Check sheet for the modelled part. Datum: model origin and axes. Units: mm. Face numbers are marked on the shaded views. A direction names the side the tool comes from. Coordinates: 2 decimals unless noted, no trailing zeros. Order: outer loops, then holes, each group sorted by start corner. A loop starts at its lowest first (then second) coordinate and runs counter-clockwise, first axis right, second up.
from build123d import *

# Parameters (mm, degrees)
BOSS_EXTRUDE1_DEPTH  = 26.75
BOSS_EXTRUDE2_DEPTH  = 1.25
FILLET1_R            = 1.25
FILLET1_OF_MIRROR1_R = 1.25
SKETCH5_R            = 3
CUT_EXTRUDE1_DEPTH   = 1.25
SKETCH6_R            = 3
CUT_EXTRUDE2_DEPTH   = 1.25
CUT_EXTRUDE3_DEPTH   = 1.25
CUT_EXTRUDE4_DEPTH   = 1.25


with BuildPart() as part:
    # Sketch1 → Boss-Extrude1 (new body)
    with BuildSketch(Plane(origin=(0, 0, 0), x_dir=(0, 0, -1), z_dir=(1, 0, 0))):
        Polygon((45.443853174, 24.716321972), (-44.407308019, 15.814225038), (-85.72558755, -16.072016683), (-86.489274142, -15.082429501), (-44.887235053, 17.022795826), (45.320611525, 25.960231734), align=None)
    extrude(amount=BOSS_EXTRUDE1_DEPTH)

    # Sketch2 → Boss-Extrude2 (add)
    with BuildSketch(Plane(origin=(26.75, 0, 0), x_dir=(0, 0, -1), z_dir=(1, 0, 0))):
        Polygon((46.306544717, 16.008953638), (-41.047818784, 7.354229524), (-80.379781408, -22.999126953), (-86.489274142, -15.082429501), (-44.887235053, 17.022795826), (45.320611525, 25.960231734), align=None)
    boss_extrude2 = extrude(amount=BOSS_EXTRUDE2_DEPTH)

    # Fillet1
    fillet1_edges = [part.edges().sort_by_distance(p)[0] for p in [
        (28, 21.49151378, -0.216688236),
        (28, 0.970183162, 65.688254597),
    ]]
    fillet(fillet1_edges, radius=FILLET1_R)

    # Mirror1: Boss-Extrude2 across plane
    add(boss_extrude2.mirror(Plane(origin=(13.375, 0, 0), x_dir=(0, 0, 1), z_dir=(1, 0, 0))))

    # Fillet1 of Mirror1
    fillet1_of_mirror1_edges = [part.edges().sort_by_distance(p)[0] for p in [
        (-1.25, 21.49151378, -0.216688236),
        (-1.25, 0.970183162, 65.688254597),
    ]]
    fillet(fillet1_of_mirror1_edges, radius=FILLET1_OF_MIRROR1_R)

    # Sketch5 → Cut-Extrude1 (cut)
    with BuildSketch(Plane(origin=(0, 21.261342533, 2.106489551), x_dir=(1, 0, 0), z_dir=(0, 0.9951278095775022, 0.09859331927408967))):
        with Locations(Location((5.55625, 41.309306291, 0), (0, 0, 270))):
            Circle(SKETCH5_R)
        with Locations(Location((21.19375, 41.309306291, 0), (0, 0, 270))):
            Circle(SKETCH5_R)
    extrude(amount=-CUT_EXTRUDE1_DEPTH, mode=Mode.SUBTRACT)

    # Sketch6 → Cut-Extrude2 (cut)
    with BuildSketch(Plane(origin=(0, 32.379495301, 24.987981728), x_dir=(1, 0, 0), z_dir=(0, 0.7916697451364806, 0.6109492733734446))):
        with Locations(Location((21.19375, -71.335540962, 0), (0, 0, 270))):
            Circle(SKETCH6_R)
        with Locations(Location((5.55625, -71.335540962, 0), (0, 0, 270))):
            Circle(SKETCH6_R)
        with Locations(Location((5.55625, -46.335540962, 0), (0, 0, 270))):
            Circle(SKETCH6_R)
        with Locations(Location((21.19375, -46.335540962, 0), (0, 0, 270))):
            Circle(SKETCH6_R)
    extrude(amount=-CUT_EXTRUDE2_DEPTH, mode=Mode.SUBTRACT)

    # Sketch7 → Cut-Extrude3 (cut)
    with BuildSketch(Plane(origin=(0, 21.261342533, 2.106489551), x_dir=(1, 0, 0), z_dir=(0, 0.9951278095775022, 0.09859331927408967))):
        with BuildLine():
            Line((8.875, -42.943848047), (17.875, -42.943848047))
            Line((17.875, -42.943848047), (17.875, -38.104983203))
            ThreePointArc((17.875, -38.104983203), (17.435660172, -37.044323031), (16.375, -36.604983203))
            Line((16.375, -36.604983203), (10.375, -36.604983203))
            ThreePointArc((10.375, -36.604983203), (9.314339828, -37.044323031), (8.875, -38.104983203))
            Line((8.875, -38.104983203), (8.875, -42.943848047))
        make_face()
        with BuildLine():
            Line((17.875, -23.604983203), (17.875, -15.104983203))
            Line((17.875, -15.104983203), (17.875, -13.604983203))
            ThreePointArc((17.875, -13.604983203), (17.435660172, -12.544323031), (16.375, -12.104983203))
            Line((16.375, -12.104983203), (10.375, -12.104983203))
            ThreePointArc((10.375, -12.104983203), (9.314339828, -12.544323031), (8.875, -13.604983203))
            Line((8.875, -13.604983203), (8.875, -15.104983203))
            Line((8.875, -15.104983203), (8.875, -23.604983203))
            Line((8.875, -23.604983203), (8.875, -28.604983203))
            Line((8.875, -28.604983203), (8.875, -30.104983203))
            ThreePointArc((8.875, -30.104983203), (9.314339828, -31.165643374), (10.375, -31.604983203))
            Line((10.375, -31.604983203), (16.375, -31.604983203))
            ThreePointArc((16.375, -31.604983203), (17.435660172, -31.165643374), (17.875, -30.104983203))
            Line((17.875, -30.104983203), (17.875, -28.604983203))
            Line((17.875, -28.604983203), (17.875, -23.604983203))
        make_face()
        with BuildLine():
            Line((16.375, 13.235019835), (10.375, 13.235019835))
            ThreePointArc((10.375, 13.235019835), (9.314339828, 12.795680007), (8.875, 11.735019835))
            Line((8.875, 11.735019835), (8.875, -5.604983203))
            ThreePointArc((8.875, -5.604983203), (9.314339828, -6.665643374), (10.375, -7.104983203))
            Line((10.375, -7.104983203), (16.375, -7.104983203))
            ThreePointArc((16.375, -7.104983203), (17.435660172, -6.665643374), (17.875, -5.604983203))
            Line((17.875, -5.604983203), (17.875, 11.735019835))
            ThreePointArc((17.875, 11.735019835), (17.435660172, 12.795680007), (16.375, 13.235019835))
        make_face()
    extrude(amount=-CUT_EXTRUDE3_DEPTH, mode=Mode.SUBTRACT)

    # Sketch8 → Cut-Extrude4 (cut)
    with BuildSketch(Plane(origin=(0, 32.379495301, 24.987981728), x_dir=(1, 0, 0), z_dir=(0, 0.7916697451364806, 0.6109492733734446))):
        with BuildLine():
            Line((8.875, -25.096490852), (8.875, -36.245103825))
            ThreePointArc((8.875, -36.245103825), (9.314339828, -37.305763997), (10.375, -37.745103825))
            Line((10.375, -37.745103825), (16.375, -37.745103825))
            ThreePointArc((16.375, -37.745103825), (17.435660172, -37.305763997), (17.875, -36.245103825))
            Line((17.875, -36.245103825), (17.875, -25.096490852))
            Line((17.875, -25.096490852), (8.875, -25.096490852))
        make_face()
    extrude(amount=-CUT_EXTRUDE4_DEPTH, mode=Mode.SUBTRACT)


solid = part.part
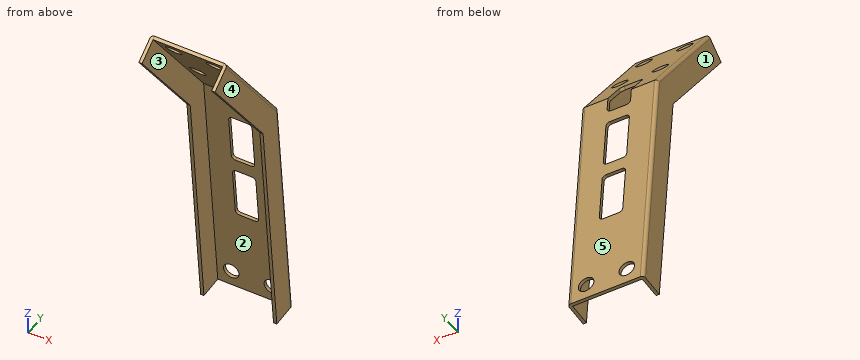
(1) Release check for a two-part mould opening along X. For the marked faces 3, 4 and 5 record: +X half, -X half, draft (parallel to the pull), parting line (faces both ways), or undercut.
Filled in:
face 3: undercut
face 4: +X half
face 5: draft
(2) Tool access check on the marked faces 1 and 2. Record the directions out of +Z, -Z, +X, -X, +Y, -Y that give a thin tool (end or side, any length) a straight path to the whole face; none if there is none.
Filled in:
face 1: +Z, -Z, -X, +Y, -Y
face 2: -Z, -Y
(3) Cross-section at B-B (x = 19.75). Enter the section's corners in (y, z), and give its area (3 significant figures).
Filled in:
outline: (-16.07, 85.73) - (-13.8, 82.78) - (-12.81, 83.54) - (-15.08, 86.49) - close; (-10.59, 78.62) - (1.47, 62.99) - (2.46, 63.75) - (-9.6, 79.38) - close; (4.69, 58.82) - (15.81, 44.41) - (23.83, -36.51) - (25.07, -36.38) - (17.02, 44.89) - (5.68, 59.59) - close; (24.35, -41.74) - (24.72, -45.44) - (25.96, -45.32) - (25.59, -41.62) - close
area: 159 mm2
(4) Go/stop test with flat-tipped pins: P1, Ø4, axis at x = 12, z = 2.5, coming from the +Y side; P2, Ø1, axis at x = 12, y = -13.5, coming from the +Z side; P3, Ø4, axis at y = 13, z = 49.5, coming from the +X side; P4, Ø3, axis at x = 18.5, y = 7.5, coming from the -Z side. Record where each tip stops, or that it passes through.
Filled in:
P1: passes through
P2: stops at z = 85.09
P3: stops at x = 28
P4: stops at z = 53.24
(5) Thickness scan on probe 1 along X at (y, z) = (17, -25); probe 2 along Z at (x, y) = (22.25, 11); probe 3 along Z at (x, y) = (1.5, 9). Record the ranges inside material, lowest first.
Filled in:
probe 1: x = -1.25 to 0, 26.75 to 28
probe 2: z = 50.65 to 52.69
probe 3: z = 53.24 to 55.28
(6) Cross-section at A-A (y = -19). Enter the section's corners in (x, z), and give its area (3 significant figures).
Filled in:
outline: (-1.25, 75.2) - (0, 75.2) - (0, 83.47) - (-1.25, 83.47) - close; (26.75, 75.2) - (28, 75.2) - (28, 83.47) - (26.75, 83.47) - close
area: 20.7 mm2
